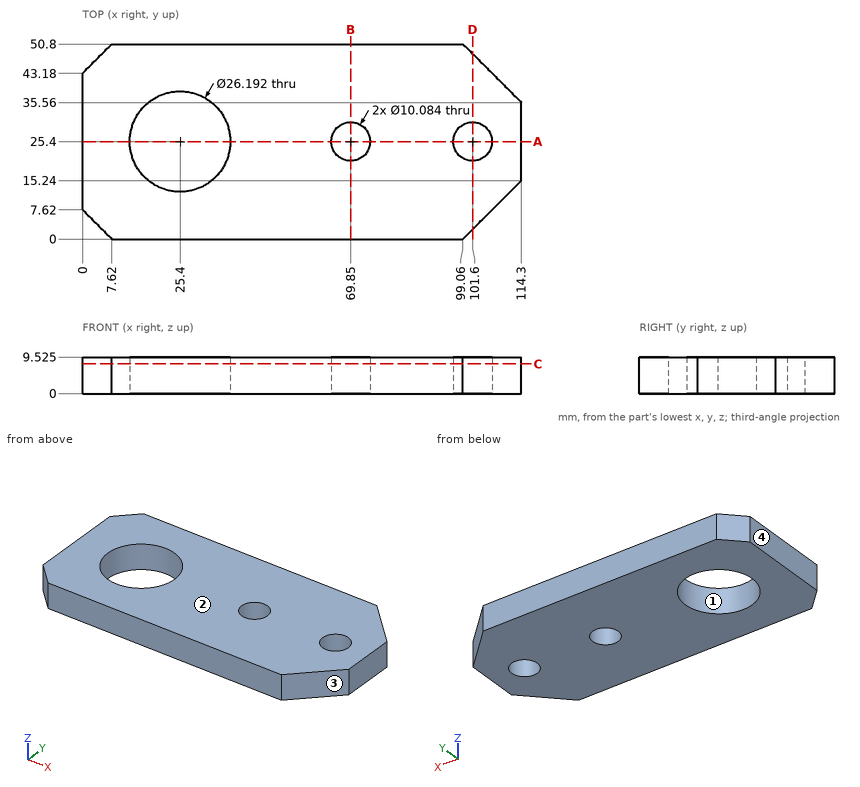
Drawing for the job (mm, zero at the part's lowest x, y, z). Give positions to 0.01 mm unless a question says otherwise; leave off trailing zeros. Write each loop counter-clockwise with the first axis right and the second up, starting at its lowest first coordinate (ties: lowest second). Pieces come first, ordered by that corner, then holes. Notation, with made-up numbers: M 2.25,-25.75 L 32.25,-25.75 A28 ccw 32.25,2.25 Z; hole C 83,-34 d7. An arc over 180 degrees is marked long. Return JSON: item names as keys, results as strings. Group by question number.
(1) Band-saw the part on D-D (x = 101.6). Give the cut face in (y, z) (1 decimal).
(2) Mould opens along X. For the marked faces 1, 2, 3 and 4 say: pulls with the +X half, pulls with the -X half, needs draft (parallel to the pull), parting line crosses it, or undercut.
(3) Band-saw the part on A-A (y = 25.4). Give the cut face in (x, z) (1 decimal), and give its area (3 significant figures).
(4) Flat gauge pin, fed straight in: pin 1 Ø2 at (y, z) = (45.5, 2) entering from -X. Where does the tip first touch, or does it go through?
(5) Band-saw the part on C-C (z = 7.75). Give the cut face in (x, y).
(6) Drill centre lines: L1, parallel to X at y = 29.5, z = 6.5 (1 decimal); L2, parallel to Y at x = 25.4, z = 3.75; L3, parallel to Y at x = 101.6, z = 6.25. Where is each one in solid material? Low to high. Write a range as [from, to].
(7) Band-saw the part on B-B (x = 69.85). Give the cut face in (y, z) (1 decimal), and give its area (3 significant figures).
Entries:
{
 "1": {"outline": "M 2.5,0 L 20.4,0 L 20.4,9.5 L 2.5,9.5 Z; M 30.4,0 L 48.3,0 L 48.3,9.5 L 30.4,9.5 Z"},
 "2": {"face 1": "undercut", "face 2": "needs draft", "face 3": "pulls with the +X half", "face 4": "pulls with the -X half"},
 "3": {"outline": "M 0,0 L 12.3,0 L 12.3,9.5 L 0,9.5 Z; M 38.5,0 L 64.8,0 L 64.8,9.5 L 38.5,9.5 Z; M 74.9,0 L 96.6,0 L 96.6,9.5 L 74.9,9.5 Z; M 106.6,0 L 114.3,0 L 114.3,9.5 L 106.6,9.5 Z", "area": "647 mm^2"},
 "4": {"pin 1": "stops at x = 1.32"},
 "5": {"outline": "M 0,7.62 L 7.62,0 L 99.06,0 L 114.3,15.24 L 114.3,35.56 L 99.06,50.8 L 7.62,50.8 L 0,43.18 Z; hole C 25.4,25.4 d26.19; hole C 69.85,25.4 d10.08; hole C 101.6,25.4 d10.08"},
 "6": {"L1": "x = [0, 13], [37.8, 66.9], [72.8, 98.7], [104.5, 114.3]", "L2": "y = [0, 12.3], [38.5, 50.8]", "L3": "y = [2.54, 20.36], [30.44, 48.26]"},
 "7": {"outline": "M 0,0 L 20.4,0 L 20.4,9.5 L 0,9.5 Z; M 30.4,0 L 50.8,0 L 50.8,9.5 L 30.4,9.5 Z", "area": "388 mm^2"}
}
